from build123d import *

# Parameters (mm, degrees)
SKETCH_1_W           = 65.5
SKETCH_1_H           = 65.5
SKETCH_1_R           = 3.6
EXTRUDE_1_DEPTH      = 3
FILLET_1_R           = 3
EXTRUDE_2_DEPTH      = 1
EXTRUDE_2_DEPTH_BACK = 11.5
SKETCH_3_R           = 3.6
SKETCH_4_R           = 7.7
EXTRUDE_3_DEPTH      = 9


with BuildPart() as part:
    # 草图1 → 凸台-拉伸1 (new body)
    with BuildSketch(Plane.XY):
        Rectangle(SKETCH_1_W, SKETCH_1_H)
        with Locations((-20, 20)):
            Circle(SKETCH_1_R, mode=Mode.SUBTRACT)
        with Locations(Location((20, 20, 0), (0, 0, 180))):
            Circle(SKETCH_1_R, mode=Mode.SUBTRACT)
        with Locations((20, -20)):
            Circle(SKETCH_1_R, mode=Mode.SUBTRACT)
        with Locations(Location((-20, -20, 0), (0, 0, 180))):
            Circle(SKETCH_1_R, mode=Mode.SUBTRACT)
        with BuildLine():
            Line((-10.15, 22.5), (10.15, 22.5))
            ThreePointArc((10.15, 22.5), (12.65, 20), (10.15, 17.5))
            Line((10.15, 17.5), (-10.15, 17.5))
            ThreePointArc((-10.15, 17.5), (-12.65, 20), (-10.15, 22.5))
        make_face(mode=Mode.SUBTRACT)
        with BuildLine():
            Line((-10.15, -22.5), (10.15, -22.5))
            ThreePointArc((10.15, -22.5), (12.65, -20), (10.15, -17.5))
            Line((10.15, -17.5), (-10.15, -17.5))
            ThreePointArc((-10.15, -17.5), (-12.65, -20), (-10.15, -22.5))
        make_face(mode=Mode.SUBTRACT)
    extrude(amount=EXTRUDE_1_DEPTH)

    # 圆角1
    fillet_1_edges = [part.edges().sort_by_distance(p)[0] for p in [
        (-32.75, 32.75, 1.5),
        (32.75, 32.75, 1.5),
        (32.75, -32.75, 1.5),
        (-32.75, -32.75, 1.5),
    ]]
    fillet(fillet_1_edges, radius=FILLET_1_R)

    # 草图3 → 凸台-拉伸2 (add, two sides: drawn at the far end of the back side and taken through both)
    with BuildSketch(Plane.XY.offset(3).offset(-EXTRUDE_2_DEPTH_BACK)):
        with Locations((-20, 20)):
            Circle(SKETCH_3_R)
        with Locations((-20, -20)):
            Circle(SKETCH_3_R)
        with Locations((20, 20)):
            Circle(SKETCH_3_R)
        with Locations((20, -20)):
            Circle(SKETCH_3_R)
    extrude(amount=EXTRUDE_2_DEPTH + EXTRUDE_2_DEPTH_BACK)

    # 草图4 → 凸台-拉伸3 (add)
    with BuildSketch(Plane(origin=(0, 0, -8.5), x_dir=(-1, 0, 0), z_dir=(0, 0, -1))):
        with Locations((-20, -20)):
            Circle(SKETCH_4_R)
        with Locations((-20, 19.85)):
            Circle(SKETCH_4_R)
        with Locations((19.85, 19.85)):
            Circle(SKETCH_4_R)
        with Locations((19.85, -20)):
            Circle(SKETCH_4_R)
    extrude(amount=EXTRUDE_3_DEPTH)


solid = part.part
Read the model definition and answer for the solid it produces. Units are mm, in the model's axes. A direction names the side the tool comes from. Give positions to 0.01 mm unless a question says otherwise; leave off trailing zeros. Write each loop counter-clockwise with the first axis right and the second up, starting at its lowest first coordinate (ties: lowest second). Pieces come first, ordered by that corner, then holes. Notation, with made-up numbers: (79.25, 15.5) - (119.25, 15.5) arc R22 ccw to (119.25, 54.5) - close; hole circle Ø10 at (7.25, 1.5). An arc over 180 degrees is marked (long way). Answer in a Markdown table with one row per item. Add a question column.
Item 1: A tool of negligible diameter and unlimited length cuts with its end or side. For faces 5 (the face through (20, 20, 4)), 6 (the face through (19.22, -23.514, 3.493)), 7 (the face through (-20.78, -23.514, -4.31)), 8 (the face through (25.68, -14.8, -12.94)), from which of +Z, -Z, +X, -X, +Y, -Y can it reach the whole face along a straight path? Write none if from no direction.
Item 2: Flat-ended cylindrical pins translate along their axes: P1, Ø3, axis at x = 6, y = -23, coming from the +Z side; P2, Ø1.5, axis at x = -7, y = -22.5, coming from the -Z side; P3, Ø10, axis at x = 24.5, y = 23, coming from the +Z side; P4, Ø6, axis at y = -25.5, z = -4, coming from the -X side. Find the tip coordinate at first contact, or state that the pin passes through.
Item 3: Determine the mould class of faces 1 (the face through (-12.65, 19.95, 1.48)), 2 (the face through (-21.5, 16.5, -8.5)), 3 (the face through (0, 32.75, 1)), 4 (the face through (-20, 20, -17.5)) for opening direction Y: pulls with the +Y half, pulls with the -Y half, needs draft (parallel to the pull), parting line crosses it, or undercut.
Item 4: Section C-C, the plane y = 25.5 is taken. Write down the section's boundary in (x, z), and give its area (3 significant figures).
Item 5: Find the intervals of material crossed by L1, parallel to Y at x = -8, z = 1.25; L2, parallel to Z at x = 12.5, y = 24.5; L3, parallel to Z at x = -20, y = 16, in increasing order.
Item 6: Section A-A, the plane x = 3 is taken. Write down the section's boundary in (y, z), and give its area (4 significant figures).
Item 7: Section D-D, the plane z = -11.75 is taken. Write down the section's boundary in (x, y).
Recorded:
| question | item | result |
|---|---|---|
| 1 | face 5 | +Z, +X, -X, +Y, -Y |
| 1 | face 6 | +Z |
| 1 | face 7 | none |
| 1 | face 8 | -Z |
| 2 | P1 | stops at z = 3 |
| 2 | P2 | stops at z = 0 |
| 2 | P3 | stops at z = 4 |
| 2 | P4 | stops at x = -22.59 |
| 3 | face 1 | undercut |
| 3 | face 2 | undercut |
| 3 | face 3 | pulls with the +Y half |
| 3 | face 4 | needs draft |
| 4 | outline | (-32.75, 0) - (32.75, 0) - (32.75, 3) - (-32.75, 3) - close; (-25.08, -17.5) - (-14.62, -17.5) - (-14.62, -8.5) - (-25.08, -8.5) - close; (14.77, -17.5) - (25.23, -17.5) - (25.23, -8.5) - (14.77, -8.5) - close |
| 4 | area | 385 mm2 |
| 5 | L1 | y = -32.75 to -22.5, -17.5 to 17.5, 22.5 to 32.75 |
| 5 | L2 | z = 0 to 3 |
| 5 | L3 | z = -17.5 to -8.5, 0 to 3 |
| 6 | outline | (-32.75, 0) - (-22.5, 0) - (-22.5, 3) - (-32.75, 3) - close; (-17.5, 0) - (17.5, 0) - (17.5, 3) - (-17.5, 3) - close; (22.5, 0) - (32.75, 0) - (32.75, 3) - (22.5, 3) - close |
| 6 | area | 166.5 mm2 |
| 7 | outline | circle Ø15.4 at (-19.85, -20); circle Ø15.4 at (-19.85, 19.85); circle Ø15.4 at (20, -20); circle Ø15.4 at (20, 19.85) |
